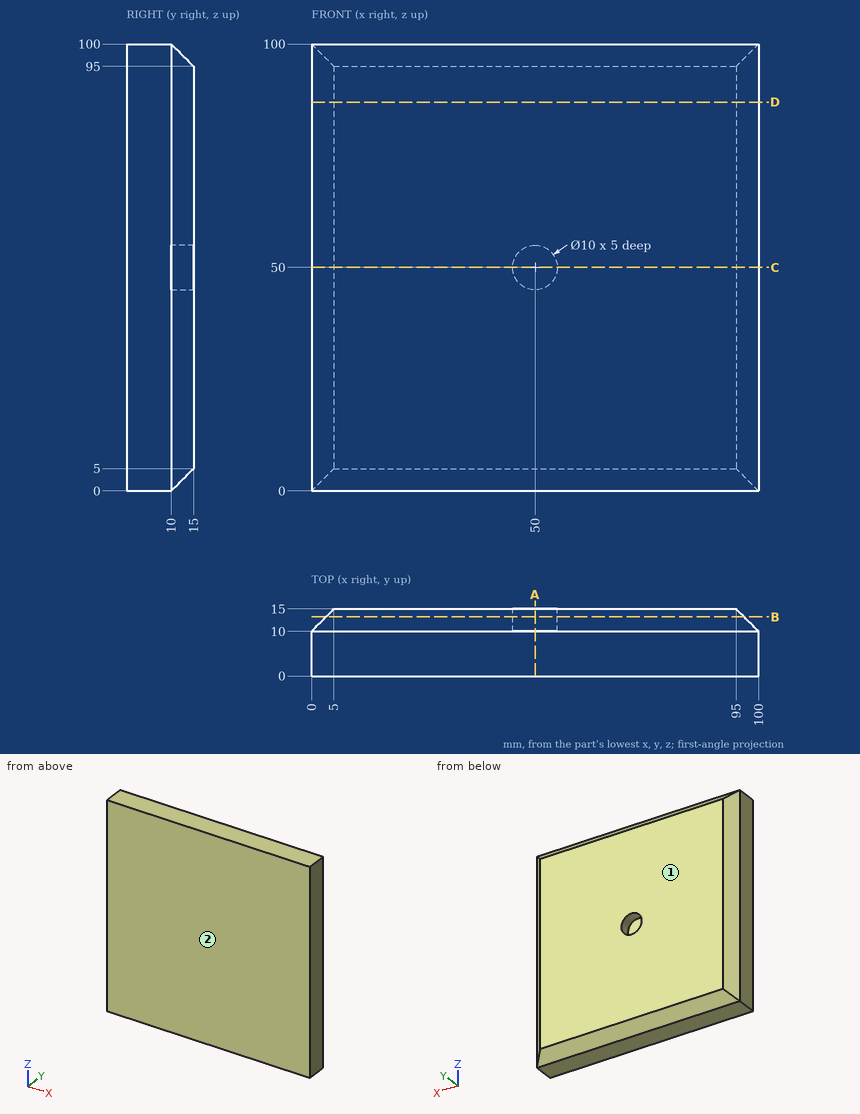
Job drawing, mm, ordinate dimensions from the low corner. One solid piece. Round coordinates to 2 decimals unless told otherwise and drop trailing zeros. Order: outer loops, then holes, each group sorted by start corner. A loop starts at its lowest first (then second) coordinate and runs counter-clockwise, first axis right, second up. Notation, with made-up numbers: (63.5, 33.25) -> (83.5, 33.25) arc R17 cw to (83.5, 43.25) -> close; hole circle Ø4 at (55.5, -17). An arc over 180 degrees is marked (long way). Answer in a Markdown table with one row per item.
1) Band-saw the part on B-B on y = 13.25. Give the cut face in (x, z).
Values:
| item | result |
|---|---|
| outline | (3.25, 3.25) -> (96.75, 3.25) -> (96.75, 96.75) -> (3.25, 96.75) -> close; hole circle Ø10 at (50, 50) |
2) Band-saw the part on D-D on z = 87. Give the cut face in (x, y).
Values:
| item | result |
|---|---|
| outline | (0, 0) -> (100, 0) -> (100, 10) -> (95, 15) -> (5, 15) -> (0, 10) -> close |
3) Band-saw the part on C-C on z = 50. Give the cut face in (x, y), and give its area (4 significant figures).
Values:
| item | result |
|---|---|
| outline | (0, 0) -> (100, 0) -> (100, 10) -> (95, 15) -> (55, 15) -> (55, 10) -> (45, 10) -> (45, 15) -> (5, 15) -> (0, 10) -> close |
| area | 1,425 mm2 |
4) Pin check, flat tips, straight feed: P1, Ø8, axis at x = 65, y = 13, coming from the +Z side; P2, Ø9, axis at x = 50, z = 50, coming from the +Y side. Stop position of each tip, or through.
Values:
| item | result |
|---|---|
| P1 | z = 100 |
| P2 | y = 10 |
5) Wall check: L1, parallel to X at y = 13.85, z = 50; L2, parallel to X at y = 12.35, z = 50; L3, parallel to Z at x = 47, y = 12. Give the ranges that are in metal, low to high.
Values:
| item | result |
|---|---|
| L1 | 3.85 to 45, 55 to 96.15 |
| L2 | 2.35 to 45, 55 to 97.65 |
| L3 | 2 to 46, 54 to 98 |
6) Band-saw the part on A-A on x = 50. Give the cut face in (y, z), and give its area (4 significant figures).
Values:
| item | result |
|---|---|
| outline | (0, 0) -> (10, 0) -> (15, 5) -> (15, 45) -> (10, 45) -> (10, 55) -> (15, 55) -> (15, 95) -> (10, 100) -> (0, 100) -> close |
| area | 1,425 mm2 |
7) Mould opens along Y. For the marked faces 1 and 2 say: released by +Y, released by -Y, zero draft, split by the parting line, or undercut.
Values:
| item | result |
|---|---|
| face 1 | released by +Y |
| face 2 | released by -Y |
